Input: dimensioned drawing with shaded views. Units: mm. Origin: part minimum x, y, z. A direction names the side the tool comes from. Coordinates: 2 decimals unless noted, no trailing zeros. Order: outer loops, then holes, each group sorted by start corner. A loop starts at its lowest first (then second) coordinate and runs counter-clockwise, first axis right, second up.
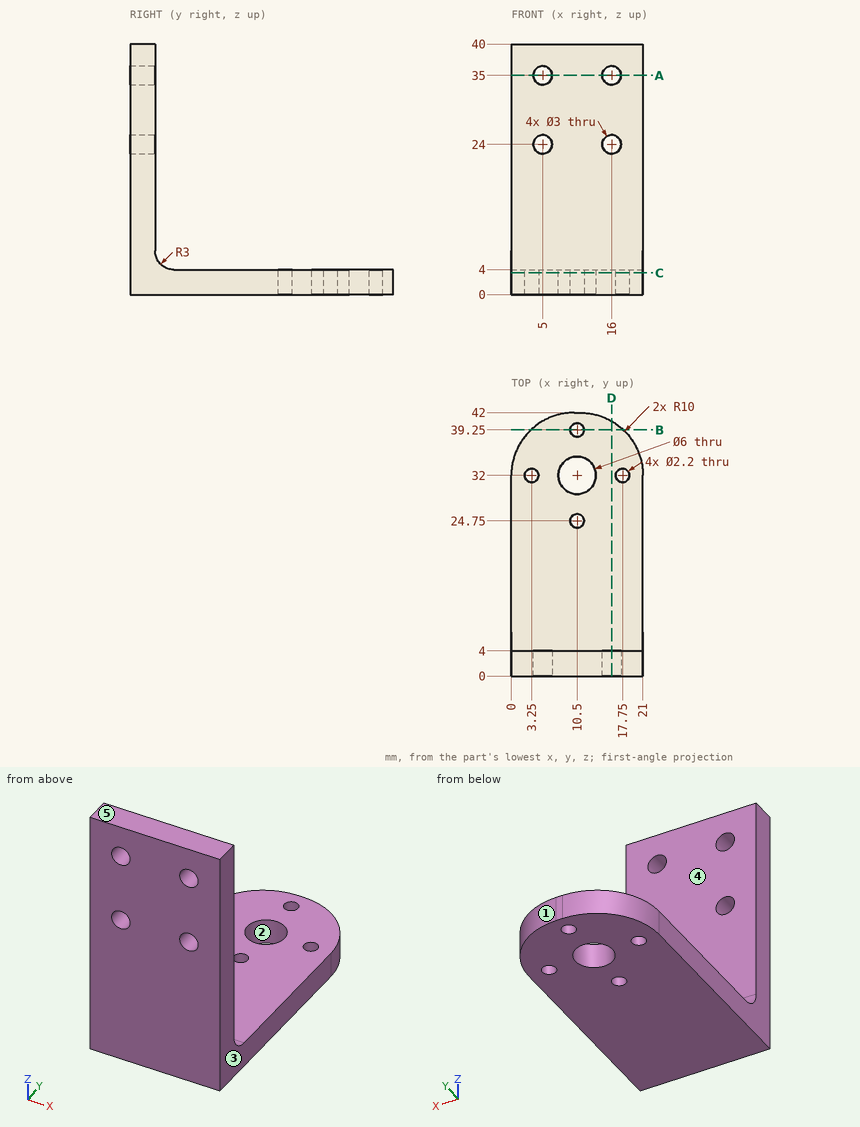
1. Access query for the marked faces 4 and 5. Directions: +Z, -Z, +X, -X, +Y, -Y. A direction counts if a zero-diameter tool reaches every point of the face in a straight line with its end or side. Return the directions, or none.
Findings:
face 4: +Z, +X, -X, +Y
face 5: +Z, +X, -X, +Y, -Y
2. Draft query along Y for the marked faces 1, 2 and 3. Return one class per face: released by +Y, released by -Y, zero draft, split by the parting line, or undercut.
Findings:
face 1: released by +Y
face 2: undercut
face 3: zero draft
3. Pin query (flat end, axial travel): P1, Ø1.8, axis at x = 16, z = 24, coming from the -Y side; P2, Ø4, axis at x = 17, z = 11.5, coming from the -Y side; P3, Ø6, axis at x = 4, y = 25, coming from the +Z side; P4, Ø4, axis at x = 5, z = 24, coming from the +Y side. Return the tip coordinate at first contact, or that it passes through.
Findings:
P1: passes through
P2: stops at y = 0
P3: stops at z = 4
P4: stops at y = 4
4. Section query B-B on y = 39.25. Return loops of the section in (x, z), plus the area to 3 significant figures.
Findings:
outline: (3.11, 0) - (9.4, 0) - (9.4, 4) - (3.11, 4) - close; (11.6, 0) - (17.89, 0) - (17.89, 4) - (11.6, 4) - close
area: 50.3 mm2
5. Section query A-A on z = 35. Return loops of the section in (x, y).
Findings:
outline: (0, 0) - (3.5, 0) - (3.5, 4) - (0, 4) - close; (6.5, 0) - (14.5, 0) - (14.5, 4) - (6.5, 4) - close; (17.5, 0) - (21, 0) - (21, 4) - (17.5, 4) - close
6. Section query C-C on z = 3.5. Return loops of the section in (x, y), plus the area to 3 significant figures.
Findings:
outline: (0, 0) - (21, 0) - (21, 32) arc R10 ccw to (11, 42) - (10, 42) arc R10 ccw to (0, 32) - close; hole circle Ø2.2 at (3.25, 32); hole circle Ø6 at (10.5, 32); hole circle Ø2.2 at (10.5, 24.75); hole circle Ø2.2 at (10.5, 39.25); hole circle Ø2.2 at (17.75, 32)
area: 796 mm2
7. Ray query, line 1 (X direction, y = 1.65, z = 35); line 2 (X direction, y = 32, z = 3); line 3 (Z direction, x = 16, y = 1.5). Return the intervals inside material, ascending.
Findings:
line 1: x = 0 to 3.5, 6.5 to 14.5, 17.5 to 21
line 2: x = 0 to 2.15, 4.35 to 7.5, 13.5 to 16.65, 18.85 to 21
line 3: z = 0 to 22.5, 25.5 to 33.5, 36.5 to 40
8. Section query D-D on x = 16. Return loops of the section in (y, z), plus the area to 3 significant figures.
Findings:
outline: (0, 0) - (40.66, 0) - (40.66, 4) - (7, 4) arc R3 cw to (4, 7) - (4, 22.5) - (0, 22.5) - close; (0, 25.5) - (4, 25.5) - (4, 33.5) - (0, 33.5) - close; (0, 36.5) - (4, 36.5) - (4, 40) - (0, 40) - close
area: 285 mm2
